```python
from build123d import *

# Parameters (mm, degrees)
TUBE_R             = 45
TUBE_R_2           = 43.2
TUBE_DEPTH         = 60
SKETCH_R           = 2
POCKET_DEPTH       = 326.425946
POCKET_DEPTH_BACK  = 326.425946
POLARPATTERN_COUNT = 4
SKETCH003_R        = 15
POCKET001_DEPTH    = 63.64061


with BuildPart() as part:
    # Tube → Tube (new body)
    with BuildSketch(Plane.XY):
        Circle(TUBE_R)
        Circle(TUBE_R_2, mode=Mode.SUBTRACT)
    extrude(amount=TUBE_DEPTH)

    # Sketch → Pocket (cut, two sides)
    with BuildSketch(Plane.XZ) as pocket_sk:
        with Locations((0, 10)):
            Circle(SKETCH_R)
    pocket = extrude(amount=-POCKET_DEPTH, mode=Mode.SUBTRACT) + extrude(pocket_sk.sketch, amount=POCKET_DEPTH_BACK, mode=Mode.SUBTRACT)

    # PolarPattern: Pocket ×4 about axis
    polarpattern_axis = Axis((0, 0, 0), (0, 0, 1))
    for i in range(1, POLARPATTERN_COUNT):
        add(pocket.rotate(polarpattern_axis, i * 360 / POLARPATTERN_COUNT), mode=Mode.SUBTRACT)

    # Sketch003 → Pocket001 (cut, through all)
    with BuildSketch(Plane(origin=(0, 0, 0), x_dir=(-0.707107, -0.707107, 0), z_dir=(-0.707107, 0.707107, 0))):
        with Locations((0, 25)):
            Circle(SKETCH003_R)
    extrude(amount=-POCKET001_DEPTH, mode=Mode.SUBTRACT)


solid = part.part
```
The model under review builds one solid part; all positions refer to its coordinate system, in mm. Round coordinates to 2 decimals unless told otherwise and drop trailing zeros. Loops run counter-clockwise (first coordinate to the right, second up) from the corner with the lowest first, then second, coordinate; pieces in that order, holes last.
1) Consider section C-C on y = 23.5. State the section outline as (x, z) points, then the cut area to 3 significant figures.
Values follow:
outline: (-38.38, 0) - (-36.25, 0) - (-36.25, 60) - (-38.38, 60) - close; (36.25, 0) - (38.38, 0) - (38.38, 60) - (36.25, 60) - close
area: 255 mm2
2) Consider section D-D on z = 4. State the section outline as (x, y) points.
Values follow:
outline: circle Ø90 at (0, 0); hole circle Ø86.4 at (0, 0)
3) Clearance check with flat-ended pins moving along their axes: P1, Ø8, axis at y = -24.5, z = 53.5, coming from the -X side; P2, Ø4, axis at x = 3, z = 22, coming from the -Y side; P3, Ø12, axis at y = -26, z = 12, coming from the +X side. State where each tip first meets the part, or that it passes through.
Values follow:
P1: stops at x = -40.06
P2: stops at y = -44.99
P3: stops at x = 40.31
4) Wall thickness on line 1 along X through (y, z) = (0, 45); line 2 along Z through (x, y) = (44.45, 0): over which ranges is each line inside the solid? List them lowest first.
Values follow:
line 1: x = -45 to -43.2, 43.2 to 45
line 2: z = 0 to 8, 12 to 60
5) Consider section A-A on y = 0. State the section outline as (x, z) points, then the cut area to 3 significant figures.
Values follow:
outline: (-45, 0) - (-43.2, 0) - (-43.2, 8) - (-45, 8) - close; (-45, 12) - (-43.2, 12) - (-43.2, 60) - (-45, 60) - close; (43.2, 0) - (45, 0) - (45, 8) - (43.2, 8) - close; (43.2, 12) - (45, 12) - (45, 60) - (43.2, 60) - close
area: 202 mm2
6) The part is to be moulded in two halves that separate along X. For faces 1 (the face through (-33.17, 30.41, 29.58)), 2 (the face through (-17, 40, 0)), 3 (the face through (0, -44, 12)), 4 (the face through (33.215, -28.617, 10.357)), say which applies: pulls with the +X half, pulls with the -X half, needs draft (parallel to the pull), parting line crosses it, or undercut.
Values follow:
face 1: parting line crosses it
face 2: needs draft
face 3: undercut
face 4: undercut
